from build123d import *

# Parameters (mm, degrees)
SKETCH2_R           = 6.806368693
BOSS_EXTRUDE1_DEPTH = 6
CUT_EXTRUDE1_DEPTH  = 49
SKETCH5_W           = 0.469385106
SKETCH5_H           = 0.019240939
SKETCH5_W_2         = 0.618798201
SKETCH5_W_3         = 0.526460496
SKETCH7_R           = 0.854461161
CUT_EXTRUDE2_DEPTH  = 10


with BuildPart() as part:
    # Sketch2 → Boss-Extrude1 (new body)
    with BuildSketch(Plane.XY.offset(-44.302178105)):
        with Locations((-124.156373602, -50.798156381)):
            Circle(SKETCH2_R)
    extrude(amount=-BOSS_EXTRUDE1_DEPTH)

    # Sketch3 → Revolve1 (revolve)
    with BuildSketch(Plane.ZY.offset(124.156373602), mode=Mode.PRIVATE) as revolve1_sk:
        Polygon((-44.302178105, -50.798156381), (6.183197751, -50.798156381), (6.183197751, -44.024347355), (5.148759689, -44.024347355), (5.148759689, -49.48766214), (-5.538916802, -47.052727869), (-44.302178105, -47.052727869), align=None)
    revolve(revolve1_sk.sketch.rotate(Axis((-124.156373602, -50.798156381, -44.302178105), (0, 0, 1)), 90), axis=Axis((-124.156373602, -50.798156381, -44.302178105), (0, 0, 1)))

    # Sketch4 → Cut-Extrude1 (cut)
    with BuildSketch(Plane(origin=(0, 0, 5.148759689), x_dir=(-1, 0, 0), z_dir=(0, 0, -1))):
        with BuildLine():
            ThreePointArc((122.898541187, -50.430389102), (123.18629962, -49.917048201), (123.669679719, -49.581388441))
            Line((123.669679719, -49.581388441), (123.669679719, -46.278106739))
            ThreePointArc((123.669679719, -46.278106739), (120.899785056, -47.626035521), (119.625097078, -50.430389102))
            Line((119.625097078, -50.430389102), (122.898541187, -50.430389102))
        make_face()
        with BuildLine():
            Line((124.524140881, -46.266879857), (124.524140881, -49.540323966))
            ThreePointArc((124.524140881, -49.540323966), (125.037481781, -49.828082399), (125.373141541, -50.311462498))
            Line((125.373141541, -50.311462498), (128.676423243, -50.311462498))
            ThreePointArc((128.676423243, -50.311462498), (127.328494461, -47.541567835), (124.524140881, -46.266879857))
        make_face()
        with BuildLine():
            Line((128.687650125, -51.16592366), (125.414206016, -51.16592366))
            ThreePointArc((125.414206016, -51.16592366), (125.126447583, -51.67926456), (124.643067484, -52.01492432))
            Line((124.643067484, -52.01492432), (124.643067484, -55.318206023))
            ThreePointArc((124.643067484, -55.318206023), (127.412962147, -53.97027724), (128.687650125, -51.16592366))
        make_face()
        with BuildLine():
            ThreePointArc((123.788606323, -52.055988795), (123.275265422, -51.768230362), (122.939605662, -51.284850263))
            Line((122.939605662, -51.284850263), (119.63632396, -51.284850263))
            ThreePointArc((119.63632396, -51.284850263), (120.984252742, -54.054744926), (123.788606323, -55.329432904))
            Line((123.788606323, -55.329432904), (123.788606323, -52.055988795))
        make_face()
    extrude(amount=CUT_EXTRUDE1_DEPTH, mode=Mode.SUBTRACT)

    # Sketch5 → Cut-Revolve2 (revolve, cut)
    with BuildSketch(Plane.ZY.offset(124.156373602), mode=Mode.PRIVATE) as cut_revolve2_sk:
        with Locations((-45.635234776, -44.001408158)):
            Rectangle(SKETCH5_W, SKETCH5_H)
        with Locations((-46.992779005, -44.001408158)):
            Rectangle(SKETCH5_W_2, SKETCH5_H)
        with Locations((-48.389416848, -44.001408158)):
            Rectangle(SKETCH5_W_3, SKETCH5_H)
    revolve(cut_revolve2_sk.sketch.rotate(Axis((-124.156373602, -50.798156381, -50.302178105), (0, 0, 1)), 270), axis=Axis((-124.156373602, -50.798156381, -50.302178105), (0, 0, 1)), mode=Mode.SUBTRACT)

    # Sketch7 → Cut-Extrude2 (cut)
    with BuildSketch(Plane(origin=(0, -50.430389102, 0), x_dir=(1, 0, 0), z_dir=(0, 1, 0))):
        with Locations(Location((-123.669679719, -2.475298292, 0), (0, 0, 98.000581908))):
            Circle(SKETCH7_R)
    extrude(amount=-CUT_EXTRUDE2_DEPTH, mode=Mode.SUBTRACT)


solid = part.part
Can you work these out from the model? Positions are in its coordinate system, mm. A direction names the side the tool comes from. Coordinates: 2 decimals unless noted, no trailing zeros. Order: outer loops, then holes, each group sorted by start corner. A loop starts at its lowest first (then second) coordinate and runs counter-clockwise, first axis right, second up. Notation, with made-up numbers: M -5,-33.75 L 50,-33.75 A21 ccw 50,-9.75 Z; hole C -29.5,43.5 d10. An arc over 180 degrees is marked long. Answer as CSV lines item,"result".
(1) Suppose I cut it at C-C on z = -35. Please give me the cut outline in (x, y), plus the area to 3 significant figures.
Geometry check:
outline,"M -127.88,-51.17 L -125.41,-51.17 A1.31 ccw -124.64,-52.01 L -124.64,-54.51 A3.75 ccw -123.79,-54.53 L -123.79,-52.06 A1.31 ccw -122.94,-51.28 L -120.44,-51.28 A3.75 ccw -120.43,-50.43 L -122.9,-50.43 A1.31 ccw -123.67,-49.58 L -123.67,-47.08 A3.75 ccw -124.52,-47.07 L -124.52,-49.54 A1.31 ccw -125.37,-50.31 L -127.87,-50.31 A3.75 ccw Z"
area,"13.8 mm^2"
(2) Suppose I cut it at D-D on z = -5. Please give me the cut outline in (x, y).
Geometry check:
outline,"M -127.76,-51.17 L -125.41,-51.17 A1.31 ccw -124.64,-52.01 L -124.64,-54.39 A3.62 ccw -123.79,-54.4 L -123.79,-52.06 A1.31 ccw -122.94,-51.28 L -120.57,-51.28 A3.62 ccw -120.55,-50.43 L -122.9,-50.43 A1.31 ccw -123.67,-49.58 L -123.67,-47.21 A3.62 ccw -124.52,-47.19 L -124.52,-49.54 A1.31 ccw -125.37,-50.31 L -127.75,-50.31 A3.62 ccw Z"
(3) On a 3-axis mill with a long thin cutter (end or side, diameter ignored), from which of +Z, -Z, +X, -X, +Y, -Y can I reach the whole of each face in a straight line? I mean faces 1 (the flat face through (-123.789, -53, -21)), 2 (the flat face through (-127, -50.311, -19)), 3 (the flat face through (-127, -51.166, -19)). Say none if no direction works.
Geometry check:
face 1,"+X, -Y"
face 2,"-X, +Y"
face 3,"-X, -Y"
(4) Please list where these lines run through material, in increasing order: L1, parallel to Z at x = -123, y = -45.5; L2, parallel to Z at x = -122.5, y = -49.5; L3, parallel to Y at x = -121.75, z = -15.
Geometry check:
L1,"-50.3 to -44.3, 5.15 to 6.18"
L2,"-50.3 to -43.85, 5.15 to 6.18"
L3,"-51.28 to -50.43"
(5) I'm going to push flat-ended pins straight in: pin 1 (2.5 mm diameter, centred on x = -122, z = -9.5, fed in from +Y); pin 2 (2.5 mm diameter, centred on x = -123.67, z = 2.48, fed in from +Y); pin 3 (1.5 mm diameter, centred on y = -55, z = -12, fed in from -X). Where does each tip first touch, or does it pass through?
Geometry check:
pin 1,"y = -49.85"
pin 2,"y = -48.61"
pin 3,"x = -124.64"
